Work out the finished part from the listing and answer in its coordinate system (mm). Face numbers are marked on the shaded views. A direction names the side the tool comes from. Coordinates: 2 decimals unless noted, no trailing zeros. Order: outer loops, then holes, each group sorted by start corner. A loop starts at its lowest first (then second) coordinate and runs counter-clockwise, first axis right, second up. Notation, with made-up numbers: (66, 58.5) - (100, 58.5) arc R8 cw to (100, 63.5) - close; hole circle Ø5 at (-5.75, 64). An arc over 180 degrees is marked (long way). Answer as a JSON object with one key per item and string values. Group by question number.
1) Section B-B (z = 14.75) is taken. Count the separate pieces of the cut face and the enclosed holes in it, plus the area to 3 significant figures.
2) A tool of negligible diameter and unlimited length cuts with its end or side. For the marked faces 4, 5, 6 and 7, from which of +Z, -Z, +X, -X, +Y, -Y can it reach the whole face along a straight path? Write none if from no direction.
3) Section A-A (y = -45) is taken. Give the vertices of the cut face in (x, z), plus the area to 3 significant figures.
4) The mould has two halves that part along Y. Classify the marked faces 1, 2 and 3: released by +Y, released by -Y, zero draft, split by the parting line, or undercut.
5) Section C-C (y = -35) is taken. Give the vertices of the cut face in (x, z), plus the area to 3 significant figures.
6) Each of these flat-tipped pins is pushed along its axis until it touches: P1, Ø5, axis at y = -30, z = 12, coming from the -X side; P2, Ø6.5, axis at x = 21.5, y = -36, coming from the +Z side; P3, Ø8, axis at y = -16, z = 14.5, coming from the +X side. Where does it stop, or does it pass through?
7) Find the intervals of material crossed by line 1 along Y through (x, z) = (7.75, 3); line 2 along X through (y, z) = (-36, 11); line 3 along Z through (x, y) = (3.75, -30), in increasing order.
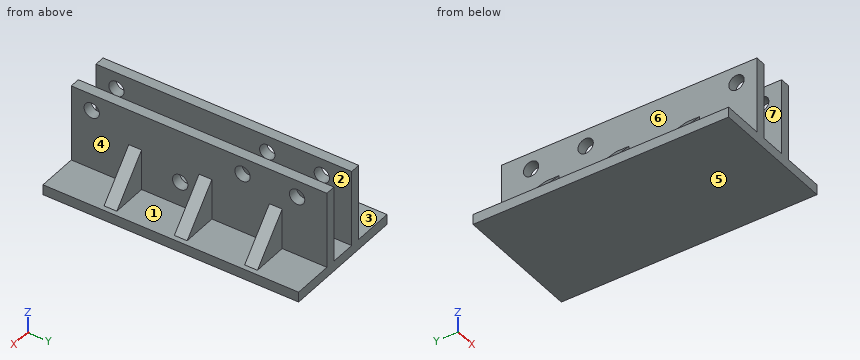
from build123d import *

# Parameters (mm, degrees)
F0_W     = 2
F0_H     = 15
F1_DEPTH = 50
F2_W     = 8
F2_H     = 2.5
F3_DEPTH = 15
F5_DEPTH = 100
F7_DEPTH = 34.4
F8_R     = 1.5
F9_DEPTH = 9


with BuildPart() as f1:
    # F0 (on Front) → F1 (new body)
    with BuildSketch(Plane.XZ):
        Polygon((12.5, 2), (12.5, 1), (15, 2), align=None)
        Polygon((0, 2), (0, 0), (10, 0), (12.5, 1), (10, 2), (8, 2), align=None)
        with Locations((9, 9.5)):
            Rectangle(F0_W, F0_H)
        Polygon((10, 2), (12.5, 1), (12.5, 2), align=None)
        Polygon((12.5, 1), (15, 0), (15, 2), align=None)
        with Locations((16, 9.5)):
            Rectangle(F0_W, F0_H)
        Polygon((15, 2), (15, 0), (25, 0), (25, 2), (17, 2), align=None)
        Polygon((12.5, 1), (10, 0), (15, 0), align=None)
    extrude(amount=F1_DEPTH)

    # F2 (on face) → F3 (join, through all)
    with BuildSketch(Plane.XY.offset(2)):
        Polygon((21, -11.25), (25, -11.25), (25, -8.75), (17, -8.75), (17, -11.25), align=None)
        Polygon((17, -25), (25, -25), (25, -23.75), (25, -22.5), (17, -22.5), align=None)
        Polygon((25, -36.25), (21, -36.25), (17, -36.25), (17, -38.75), (25, -38.75), align=None)
        Polygon((0, -25), (8, -25), (8, -22.5), (0, -22.5), (0, -23.75), align=None)
        Polygon((0, -36.25), (0, -38.75), (8, -38.75), (8, -36.25), (4, -36.25), align=None)
        with Locations((4, -10)):
            Rectangle(F2_W, F2_H)
    extrude(amount=F3_DEPTH)

    # F4 (on face) → F5 (cut)
    with BuildSketch(Plane.XZ.offset(38.75)):
        Polygon((0, 17), (0, 2), (1, 2), (8, 10), (8, 17), align=None)
    extrude(amount=-F5_DEPTH, mode=Mode.SUBTRACT)

    # F6 (on face) → F7 (cut)
    with BuildSketch(Plane.XZ.offset(38.75)):
        Polygon((17, 10), (24, 2), (25, 2), (25, 17), (17, 17), align=None)
    extrude(amount=-F7_DEPTH, mode=Mode.SUBTRACT)

    # F8 (on face) → F9 (cut, through all)
    with BuildSketch(Plane.YZ.offset(17)):
        with BuildLine():
            Line((-46.0029848111, 13.7437408806), (-44.5029848111, 13.7437408806))
            ThreePointArc((-44.5029848111, 13.7437408806), (-46.0029848111, 15.2437408806), (-47.5029848111, 13.7437408806))
            Line((-47.5029848111, 13.7437408806), (-46.0029848111, 13.7437408806))
        make_face()
        with BuildLine():
            ThreePointArc((-47.5029848111, 13.7437408806), (-46.0029848111, 12.2437408806), (-44.5029848111, 13.7437408806))
            Line((-44.5029848111, 13.7437408806), (-46.0029848111, 13.7437408806))
            Line((-46.0029848111, 13.7437408806), (-47.5029848111, 13.7437408806))
        make_face()
        with BuildLine():
            ThreePointArc((-4.3291251771, 13.7437408806), (-5.8291251771, 15.2437408806), (-7.3291251771, 13.7437408806))
            Line((-7.3291251771, 13.7437408806), (-4.3291251771, 13.7437408806))
        make_face()
        with BuildLine():
            Line((-4.3291251771, 13.7437408806), (-7.3291251771, 13.7437408806))
            ThreePointArc((-7.3291251771, 13.7437408806), (-5.8291251771, 12.2437408806), (-4.3291251771, 13.7437408806))
        make_face()
        with BuildLine():
            ThreePointArc((-15.0014732629, 13.7437408806), (-16.5014732629, 15.2437408806), (-18.0014732629, 13.7437408806))
            Line((-18.0014732629, 13.7437408806), (-16.5014732629, 13.7437408806))
            Line((-16.5014732629, 13.7437408806), (-15.0014732629, 13.7437408806))
        make_face()
        with BuildLine():
            Line((-16.5014732629, 13.7437408806), (-18.0014732629, 13.7437408806))
            ThreePointArc((-18.0014732629, 13.7437408806), (-16.5014732629, 12.2437408806), (-15.0014732629, 13.7437408806))
            Line((-15.0014732629, 13.7437408806), (-16.5014732629, 13.7437408806))
        make_face()
        with Locations((-28.6963357897, 6.7545174172)):
            Circle(F8_R)
    extrude(amount=-F9_DEPTH, mode=Mode.SUBTRACT)


solid = f1.part
Report:
{
 "1": {"separate pieces": "8", "enclosed holes": "0", "area": "173 mm²"},
 "2": {"face 4": "+Z, +X", "face 5": "-Z, +X, -X, +Y, -Y", "face 6": "+Z, -X", "face 7": "+Z, +Y, -Y"},
 "3": {"outline": "(0, 0) - (25, 0) - (25, 2) - (17, 2) - (17, 12.63) - (15, 12.63) - (15, 2) - (10, 2) - (10, 12.63) - (8, 12.63) - (8, 2) - (0, 2) - close; (8, 14.86) - (10, 14.86) - (10, 17) - (8, 17) - close; (15, 14.86) - (17, 14.86) - (17, 17) - (15, 17) - close", "area": "101 mm²"},
 "4": {"face 1": "undercut", "face 2": "zero draft", "face 3": "undercut"},
 "5": {"outline": "(0, 0) - (25, 0) - (25, 2) - (17, 2) - (17, 17) - (15, 17) - (15, 2) - (10, 2) - (10, 17) - (8, 17) - (8, 2) - (0, 2) - close", "area": "110 mm²"},
 "6": {"P1": "stops at x = 8", "P2": "stops at z = 8.56", "P3": "stops at x = 17"},
 "7": {"line 1": "y = -38.75 to -36.25, -25 to -22.5, -11.25 to -8.75", "line 2": "x = 8 to 10, 15 to 17", "line 3": "z = 0 to 2"}
}
